Build history of the part. All positions in model axes, mm. A direction names the side the tool comes from. Give positions to 0.01 mm unless a question says otherwise; leave off trailing zeros. Order: outer loops, then holes, each group sorted by start corner. A loop starts at its lowest first (then second) coordinate and runs counter-clockwise, first axis right, second up. Notation, with made-up numbers: (88.25, 61.5) - (104.25, 61.5) arc R21 ccw to (104.25, 68.5) - close; hole circle Ø8 at (11, -21). An arc over 180 degrees is marked (long way). Use a Markdown table: item, result.
from build123d import *

# Parameters (mm, degrees)
SKETCH1_R           = 2
BOSS_EXTRUDE1_DEPTH = 4
SKETCH2_R           = 7
BOSS_EXTRUDE2_DEPTH = 5
BOSS_EXTRUDE6_DEPTH = 40
BOSS_EXTRUDE7_DEPTH = 4
SKETCH9_W           = 30
SKETCH9_H           = 4
BOSS_EXTRUDE8_DEPTH = 200


with BuildPart() as part:
    # Sketch1 → Boss-Extrude1 (new body)
    with BuildSketch(Plane(origin=(0, 0, 0), x_dir=(1, 0, 0), z_dir=(0, 1, 0))):
        with BuildLine():
            Line((1, -41.732050808), (35.641016151, -21.732050808))
            Line((35.641016151, -21.732050808), (32.641016151, -16.535898385))
            ThreePointArc((32.641016151, -16.535898385), (24.260749779, -13.277014078), (20, -5.358983849))
            Line((20, -5.358983849), (20, 20))
            Line((20, 20), (-14, 20))
            Line((-14, 20), (-24.606601718, 30.606601718))
            Line((-24.606601718, 30.606601718), (-30.606601718, 24.606601718))
            Line((-30.606601718, 24.606601718), (-20, 14))
            Line((-20, 14), (-20, -5.358983849))
            Line((-20, -5.358983849), (1, -41.732050808))
        make_face()
        with Locations(Location((-15, 15, 0), (0, 0, 270))):
            Circle(SKETCH1_R, mode=Mode.SUBTRACT)
        with Locations(Location((15, 15, 0), (0, 0, 270))):
            Circle(SKETCH1_R, mode=Mode.SUBTRACT)
        with BuildLine():
            Line((-2.645751311, -3), (2.645751311, -3))
            ThreePointArc((2.645751311, -3), (0, 4), (-2.645751311, -3))
        make_face(mode=Mode.SUBTRACT)
    extrude(amount=BOSS_EXTRUDE1_DEPTH)

    # Sketch2 → Boss-Extrude2 (add)
    with BuildSketch(Plane(origin=(0, 4, 0), x_dir=(1, 0, 0), z_dir=(0, 1, 0))):
        with Locations(Location((0, 0, 0), (0, 0, 270))):
            Circle(SKETCH2_R)
        with BuildLine():
            Line((-2.645751311, -3), (2.645751311, -3))
            ThreePointArc((2.645751311, -3), (0, 4), (-2.645751311, -3))
        make_face(mode=Mode.SUBTRACT)
    extrude(amount=BOSS_EXTRUDE2_DEPTH)

    # Sketch7 → Boss-Extrude6 (add)
    with BuildSketch(Plane.XZ):
        Polygon((1, 41.732050808), (35.641016151, 21.732050808), (33.641016151, 18.267949192), (-1, 38.267949192), align=None)
    extrude(amount=BOSS_EXTRUDE6_DEPTH)

    # Sketch8 → Boss-Extrude7 (add)
    with BuildSketch(Plane.XZ.offset(40)):
        Polygon((50.641016151, 46.558112383), (65.641016151, 20.577350269), (35.641016151, 21.732050808), (1, 41.732050808), align=None)
    extrude(amount=-BOSS_EXTRUDE7_DEPTH)

    # Sketch9 → Boss-Extrude8 (add)
    with BuildSketch(Plane(origin=(58.141016151, 0, 33.567731326), x_dir=(0.5000000000000051, 0, -0.8660254037844357), z_dir=(0.8660254037844357, 0, 0.5000000000000051))):
        with Locations((0, -38)):
            Rectangle(SKETCH9_W, SKETCH9_H)
    extrude(amount=BOSS_EXTRUDE8_DEPTH)


solid = part.part
1) Slice it at B-B (y = -23). Write the cut outline in (x, z), and give its area (3 significant figures).
Computed:
| item | result |
|---|---|
| outline | (-1, 38.27) - (33.64, 18.27) - (35.64, 21.73) - (1, 41.73) - close |
| area | 160 mm² |
2) Two-plate mould, pull along X, no slides. Class faces 4 (the cylindrical face through (0, 4, -4)), 5 (the flat face through (0, 4, 3)), 6 (the cylindrical face through (-6.834, 6.465, -1.517)), 7 (the cylindrical face through (24.4, 2, 13.4)): +X half, -X half, draft (parallel to the pull), parting line (faces both ways), or undercut.
Computed:
| item | result |
|---|---|
| face 4 | undercut |
| face 5 | undercut |
| face 6 | parting line |
| face 7 | +X half |
3) Slice it at A-A (z = 0). Write the cut outline in (x, y), and give its area (3 significant figures).
Computed:
| item | result |
|---|---|
| outline | (-20, 0) - (-4, 0) - (-4, 9) - (-7, 9) - (-7, 4) - (-20, 4) - close; (4, 0) - (20, 0) - (20, 4) - (7, 4) - (7, 9) - (4, 9) - close |
| area | 158 mm² |
4) Tool access for faces 1 (the flat face through (16.56, -19.72, 28.13)), 2 (the flat face through (151.031, -38.028, 69.877)), 3 (the flat face through (18.08, -15.72, 31.87)): list every direction of +Z, -Z, +X, -X, +Y, -Y with a clear straight run to the whole face (end or side of a thin tool).
Computed:
| item | result |
|---|---|
| face 1 | -Z, -X, -Y |
| face 2 | -Z, +X, +Y, -Y |
| face 3 | +Z, +X, +Y |
5) Slice it at C-C (x = 77.5). Write the cut outline in (y, z), and give its area (3 significant figures).
Computed:
| item | result |
|---|---|
| outline | (-40, 27.42) - (-36, 27.42) - (-36, 62.07) - (-40, 62.07) - close |
| area | 139 mm² |
6) Slice it at D-D (z = 35). Write the cut outline in (x, y), and give its area (3 significant figures).
Computed:
| item | result |
|---|---|
| outline | (-2.89, 0) - (4.66, 0) - (4.66, -40) - (90.62, -40) - (90.62, -36) - (12.66, -36) - (12.66, 4) - (-2.89, 4) - close |
| area | 694 mm² |
7) Pin check, flat tips, straight feed: P1, Ø4.5, axis at y = 1.5, z = -1.5, coming from the +X side; P2, Ø8, axis at y = -28.5, z = 61, coming from the +X side; P3, Ø3, axis at y = 2.5, z = -6.5, coming from the -X side; P4, Ø2, axis at x = -3, y = 1, coming from the -Z side. Stop position of each tip, or through.
Computed:
| item | result |
|---|---|
| P1 | stops at x = 20 |
| P2 | passes through |
| P3 | stops at x = -20 |
| P4 | stops at z = -20 |
8) Wall check: line 1 (X direction, y = 2.4, z = -15); line 2 (X direction, y = 7, z = 0); line 3 (Y direction, x = 218.5, z = 133). Give the ranges that are in metal, low to high. Write a range as from..to.
Computed:
| item | result |
|---|---|
| line 1 | x = -21..-17, -13..13, 17..20 |
| line 2 | x = -7..-4, 4..7 |
| line 3 | y = -40..-36 |
